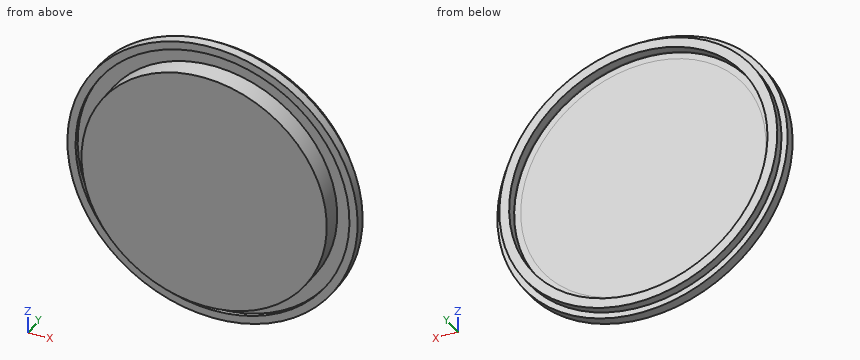
```python
from build123d import *
from build123d.topology import SkipClean

# Parameters (mm, degrees)
SKETCH_1_R          = 17
SKETCH_1_R_2        = 15.8
EXTRUDE_1_DEPTH     = 1
EXTRUDE_START       = 1.2
SKETCH_2_R          = 17.75
SKETCH_2_R_2        = 15.8
EXTRUDE_2_DEPTH     = 1.2
SKETCH_3_R          = 16.75
SKETCH_3_R_2        = 15.8
CUT_EXTRUDE_1_DEPTH = 0.5
SKETCH_4_R          = 15.8
SKETCH_4_R_2        = 15
EXTRUDE_3_DEPTH     = 0.5
SKETCH_6_R          = 15
EXTRUDE_4_DEPTH     = 3


with BuildPart() as part:
    # Sketch 1 → Extrude 1 (new body)
    with BuildSketch(Plane(origin=(0, 0, 0), x_dir=(1, 0, 0), z_dir=(0, 1, 0))):
        with Locations(Location((0, 0, 0), (0, 0, 270))):
            Circle(SKETCH_1_R)
        with Locations(Location((0, 0, 0), (0, 0, 270))):
            Circle(SKETCH_1_R_2, mode=Mode.SUBTRACT)
    extrude(amount=EXTRUDE_1_DEPTH)

    # Sketch 2 → Extrude 2 (add)
    with SkipClean():  # the faces are left unmerged after this step: merging them gives an invalid solid
        with BuildSketch(Plane.XZ.offset(EXTRUDE_START)):
            with Locations(Location((0, 0, 0), (0, 0, 270))):
                Circle(SKETCH_2_R)
            with Locations(Location((0, 0, 0), (0, 0, 270))):
                Circle(SKETCH_2_R_2, mode=Mode.SUBTRACT)
        extrude(amount=-EXTRUDE_2_DEPTH)

    # Sketch 3 → Cut-Extrude 1 (cut)
    with SkipClean():  # the faces are left unmerged after this step: merging them gives an invalid solid
        with BuildSketch(Plane(origin=(0, -1.2, 0), x_dir=(-1, 0, 0), z_dir=(0, -1, 0))):
            with Locations(Location((0, 0, 0), (0, 0, 90))):
                Circle(SKETCH_3_R)
            with Locations(Location((0, 0, 0), (0, 0, 90))):
                Circle(SKETCH_3_R_2, mode=Mode.SUBTRACT)
        extrude(amount=-CUT_EXTRUDE_1_DEPTH, mode=Mode.SUBTRACT)



with BuildPart() as body_2:
    # Sketch 4 → Extrude 3 (new body)
    with BuildSketch(Plane.XZ.offset(0.7)):
        with Locations(Location((0, 0, 0), (0, 0, 270))):
            Circle(SKETCH_4_R)
        with Locations(Location((0, 0, 0), (0, 0, 270))):
            Circle(SKETCH_4_R_2, mode=Mode.SUBTRACT)
    extrude(amount=-EXTRUDE_3_DEPTH)


with BuildPart() as part_1:
    with SkipClean():  # the faces are left unmerged after this step: merging them gives an invalid solid
        add(part.part)

        add(body_2.part)  # Extrude 4 merges body 2
        # Sketch 6 → Extrude 4 (add)
        with BuildSketch(Plane(origin=(0, -0.2, 0), x_dir=(1, 0, 0), z_dir=(0, 1, 0))):
            with Locations(Location((0, 0, 0), (0, 0, 270))):
                Circle(SKETCH_6_R)
        extrude(amount=-EXTRUDE_4_DEPTH)


solid = part_1.part
```
Design review of the part built by this model. Coordinates are the model's own, in mm. Coordinates: 2 decimals unless noted, no trailing zeros. Order: outer loops, then holes, each group sorted by start corner. A loop starts at its lowest first (then second) coordinate and runs counter-clockwise, first axis right, second up. Notation, with made-up numbers: (33.5, -16.5) - (37.5, -16.5) arc R17 ccw to (37.5, 2.5) - close; hole circle Ø6 at (57.25, -27). An arc over 180 degrees is marked (long way). One line per question, with ' | ' between items.
Q1. Clearance check with flat-ended pins moving along their axes: pin 1 Ø5 at (x, z) = (11.5, -9) entering from +Y; pin 2 Ø2 at (y, z) = (0, -8) entering from -X; pin 3 Ø1.5 at (x, y) = (-4.5, -1.5) entering from +Z; pin 4 Ø4 at (x, z) = (-3, -3.5) entering from +Y. State where each tip first meets the part, or that it passes through.
Answer key:
pin 1: stops at y = 1 | pin 2: stops at x = -16.31 | pin 3: stops at z = 17.34 | pin 4: stops at y = -0.2
Q2. To check wall thickness, follow line 1 along X through (y, z) = (-0.1, 0); line 2 along X through (y, z) = (0.75, 0); line 3 along Z through (x, y) = (-13, -1). State the ranges of each line that lie inside material, in increasing order.
Answer key:
line 1: x = -17.75 to -15.8, 15.8 to 17.75 | line 2: x = -17 to -15.8, 15.8 to 17 | line 3: z = -12.09 to -10.56, -7.48 to 7.48, 10.56 to 12.09
Q3. Consider section B-B, the plane x = 0. Give the boundary of the cut face in (y, z).
Answer key:
outline: (-3.2, -15) - (-0.7, -15) - (-0.7, -16.75) - (-1.2, -16.75) - (-1.2, -17.75) - (0, -17.75) - (0, -17) - (1, -17) - (1, -15.8) - (-0.2, -15.8) - (-0.2, 15.8) - (1, 15.8) - (1, 17) - (0, 17) - (0, 17.75) - (-1.2, 17.75) - (-1.2, 16.75) - (-0.7, 16.75) - (-0.7, 15) - (-3.2, 15) - close
Q4. Consider section A-A, the plane z = 0. Give the boundary of the cut face in (x, y).
Answer key:
outline: (-17.75, -1.2) - (-16.75, -1.2) - (-16.75, -0.7) - (-15, -0.7) - (-15, -3.2) - (15, -3.2) - (15, -0.7) - (16.75, -0.7) - (16.75, -1.2) - (17.75, -1.2) - (17.75, 0) - (17, 0) - (17, 1) - (15.8, 1) - (15.8, -0.2) - (-15.8, -0.2) - (-15.8, 1) - (-17, 1) - (-17, 0) - (-17.75, 0) - close
